```python
from build123d import *

# Parameters (mm, degrees)
F1_DEPTH = 25.4
F2_R     = 12.5138914525
F2_R_2   = 7.4979718204
F3_DEPTH = 38.1
F5_START = 30.48
F4_R     = 9.8673928173
F5_DEPTH = 2.54
F6_R     = 7.4979718204
F7_DEPTH = 38.101


with BuildPart() as f1:
    # F0 (on Front) → F1 (new body)
    with BuildSketch(Plane.XZ):
        Polygon((-9.8056579009, 14.4998570904), (0, 14.4998570904), (31.5032890067, 14.4998570904), (41.3089469075, 14.4998570904), (41.3089469075, 26.6004577279), (31.5032890067, 26.6004577279), (0, 26.6004577279), (-9.8056579009, 26.6004577279), align=None)
    extrude(amount=F1_DEPTH)

    # F2 (on Top) → F3 (join)
    with BuildSketch(Plane.XY):
        with Locations((15.3343798593, -12.7)):
            Circle(F2_R)
        with Locations((15.3343798593, -12.7)):
            Circle(F2_R_2, mode=Mode.SUBTRACT)
    extrude(amount=F3_DEPTH)

    # F4 (on Top) → F5 (cut)
    with BuildSketch(Plane.XY.offset(F5_START)):
        with Locations((15.3343798593, -12.7)):
            Circle(F4_R)
    extrude(amount=F5_DEPTH, mode=Mode.SUBTRACT)

    # F6 (on Top) → F7 (cut, through all)
    with BuildSketch(Plane.XY):
        with Locations((15.3343798593, -12.7)):
            Circle(F6_R)
    extrude(amount=F7_DEPTH, mode=Mode.SUBTRACT)


solid = f1.part
```
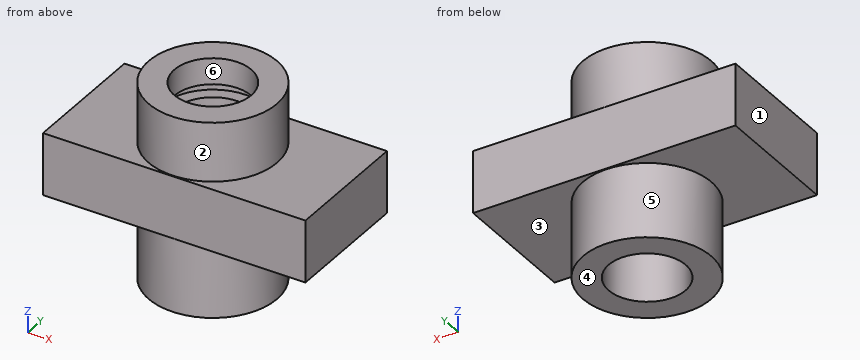
Work out the finished part from the listing and answer in its coordinate system (mm). Face numbers are marked on the shaded views. A direction names the side the tool comes from. Round coordinates to 2 decimals unless told otherwise and drop trailing zeros. Write each loop counter-clockwise with the first axis right and the second up, starting at its lowest first coordinate (ties: lowest second). Pieces come first, ordered by that corner, then holes. Notation, with made-up numbers: (30, -21) -> (88, -21) arc R29 ccw to (88, 3) -> close; hole circle Ø3 at (-32, 25.5). An arc over 180 degrees is marked (long way). Write each question's results on one line, items separated by ' | '.
1) For a pull along X with two mould halves and no side action, classify the marked faces 4, 5 and 6 as +X half, -X half, draft (parallel to the pull), parting line (faces both ways), or undercut.
Findings:
face 4: draft | face 5: parting line | face 6: undercut
2) The part is cut by section C-C (y = -4). Write down the section's boundary in (x, z).
Findings:
outline: (-9.81, 14.5) -> (6.34, 14.5) -> (6.34, 0) -> (24.33, 0) -> (24.33, 14.5) -> (41.31, 14.5) -> (41.31, 26.6) -> (24.33, 26.6) -> (24.33, 38.1) -> (6.34, 38.1) -> (6.34, 26.6) -> (-9.81, 26.6) -> close; hole (10.68, 30.48) -> (19.99, 30.48) -> (19.99, 33.02) -> (10.68, 33.02) -> close
3) The part is cut by section D-D (x = 9). Write down the section's boundary in (y, z), and give its area (3 significant figures).
Findings:
outline: (-25.4, 14.5) -> (-23.49, 14.5) -> (-23.49, 0) -> (-16.71, 0) -> (-16.71, 30.48) -> (-20.27, 30.48) -> (-20.27, 33.02) -> (-16.71, 33.02) -> (-16.71, 38.1) -> (-23.49, 38.1) -> (-23.49, 26.6) -> (-25.4, 26.6) -> close; (-8.69, 0) -> (-1.91, 0) -> (-1.91, 14.5) -> (0, 14.5) -> (0, 26.6) -> (-1.91, 26.6) -> (-1.91, 38.1) -> (-8.69, 38.1) -> (-8.69, 33.02) -> (-5.13, 33.02) -> (-5.13, 30.48) -> (-8.69, 30.48) -> close | area: 545 mm²
4) The part is cut by section A-A (y = -12.7). Write down the section's boundary in (x, z).
Findings:
outline: (-9.81, 14.5) -> (2.82, 14.5) -> (2.82, 0) -> (7.84, 0) -> (7.84, 30.48) -> (5.47, 30.48) -> (5.47, 33.02) -> (7.84, 33.02) -> (7.84, 38.1) -> (2.82, 38.1) -> (2.82, 26.6) -> (-9.81, 26.6) -> close; (22.83, 0) -> (27.85, 0) -> (27.85, 14.5) -> (41.31, 14.5) -> (41.31, 26.6) -> (27.85, 26.6) -> (27.85, 38.1) -> (22.83, 38.1) -> (22.83, 33.02) -> (25.2, 33.02) -> (25.2, 30.48) -> (22.83, 30.48) -> close
5) Consider line 1 along X through (y, z) = (-12.7, 34.35); line 2 along Z through (x, y) = (8, -15); line 3 along Z through (x, y) = (37, -1.5). Determine where each line is inside the solid, lowest interval first. Write a range as [from, to].
Findings:
line 1: x = [2.82, 7.84], [22.83, 27.85] | line 2: z = [0, 30.48], [33.02, 38.1] | line 3: z = [14.5, 26.6]
6) Which of the six approach directions +Z, -Z, +X, -X, +Y, -Y give full straight-line access (tool end or side, diameter ignored) to the marked faces 1, 2 and 3?
Findings:
face 1: +Z, -Z, -X, +Y, -Y | face 2: +Z | face 3: -Z
7) The part is cut by section B-B (z = 16). Write down the section's boundary in (x, y).
Findings:
outline: (-9.81, -25.4) -> (41.31, -25.4) -> (41.31, 0) -> (-9.81, 0) -> close; hole circle Ø15 at (15.33, -12.7)
8) A flat-ended cylindrical pin translates along its axis: pin 1 (2 mm diameter, centred on x = 30, y = -12.5, fed in from -Z). Find the tip coordinate at first contact, or state that the pin passes through.
Findings:
pin 1: stops at z = 14.5
